from build123d import *

# Parameters (mm, degrees)
EXTRUDE_1_DEPTH          = 4
CUT_EXTRUDE_1_DEPTH      = 3
CUT_EXTRUDE_2_DEPTH      = 8.071067812
CUT_EXTRUDE_2_DEPTH_BACK = 3
SKETCH_4_R               = 1
CUT_EXTRUDE_3_DEPTH      = 3


with BuildPart() as part:
    # 草圖1 → 填料-伸長1 (new body)
    with BuildSketch(Plane(origin=(0, 0, 0), x_dir=(0, 0, -1), z_dir=(1, 0, 0))):
        with BuildLine():
            Line((0, 0), (-3, 0))
            Line((-3, 0), (-3, -4))
            ThreePointArc((-3, -4), (-2.707106781, -4.707106781), (-2, -5))
            Line((-2, -5), (2, -5))
            Line((2, -5), (2, -4))
            Line((2, -4), (-1, -4))
            ThreePointArc((-1, -4), (-1.707106781, -3.707106781), (-2, -3))
            Line((-2, -3), (-2, -1))
            Line((-2, -1), (0, -1))
            Line((0, -1), (0, 0))
        make_face()
    extrude(amount=EXTRUDE_1_DEPTH)

    # 草圖2 → 除料-伸長1 (cut)
    with BuildSketch(Plane(origin=(0, 0, 0), x_dir=(1, 0, 0), z_dir=(0, 1, 0))):
        with BuildLine():
            ThreePointArc((0, -1), (0.292893219, -0.292893219), (1, 0))
            Line((1, 0), (0, 0))
            Line((0, 0), (0, -1))
        make_face()
        with BuildLine():
            Line((4, 0), (3, 0))
            ThreePointArc((3, 0), (3.707106781, -0.292893219), (4, -1))
            Line((4, -1), (4, 0))
        make_face()
    extrude(amount=-CUT_EXTRUDE_1_DEPTH, mode=Mode.SUBTRACT)

    # 草圖3 → 除料-伸長2 (cut, two sides: drawn at the far end of the back side and taken through both)
    with BuildSketch(Plane.XZ.offset(5).offset(-CUT_EXTRUDE_2_DEPTH_BACK)):
        with BuildLine():
            Line((0, -0.361789115), (0, -2))
            Line((0, -2), (2, -2))
            ThreePointArc((2, -2), (0.585786438, -1.414213562), (0, 0))
            Line((0, 0), (0, -0.361789115))
        make_face()
        with BuildLine():
            ThreePointArc((4, 0), (3.414213562, -1.414213562), (2, -2))
            Line((2, -2), (4, -2))
            Line((4, -2), (4, -0.361789115))
            Line((4, -0.361789115), (4, 0))
        make_face()
    extrude(amount=CUT_EXTRUDE_2_DEPTH + CUT_EXTRUDE_2_DEPTH_BACK, mode=Mode.SUBTRACT)

    # 草圖4 → 除料-伸長3 (cut)
    with BuildSketch(Plane.XZ.offset(5)):
        with Locations(Location((2, 0, 0), (0, 0, 270))):
            Circle(SKETCH_4_R)
    extrude(amount=-CUT_EXTRUDE_3_DEPTH, mode=Mode.SUBTRACT)


solid = part.part
The model under review builds one solid part; all positions refer to its coordinate system, in mm. A direction names the side the tool comes from. Coordinates: 2 decimals unless noted, no trailing zeros. Write each loop counter-clockwise with the first axis right and the second up, starting at its lowest first coordinate (ties: lowest second). Pieces come first, ordered by that corner, then holes. Notation, with made-up numbers: (75, -30.5) -> (123, -30.5) arc R23 ccw to (123, 3.5) -> close; hole circle Ø9 at (70, 64). An arc over 180 degrees is marked (long way). Answer in a Markdown table with one row per item.
1. We need section A-A, the plane z = 1.55. State the section outline as (x, y) points, and give its area (3 significant figures).
Answers below:
| item | result |
|---|---|
| outline | (0, -5) -> (4, -5) -> (4, -3.84) -> (0, -3.84) -> close; (0, -1) -> (4, -1) -> (4, 0) -> (0, 0) -> close |
| area | 8.66 mm^2 |
2. For faces 5 (the cylindrical face through (3.699, -0.493, 0.285)), 6 (the flat face through (3, -5, 1)), 7 (the flat face through (2, -2, 2)), list the 3-axis set-ups (+Z, -Z, +X, -X, +Y, -Y) from which the entire face can be reached by the end or side of a thin tool; tool diameter is ignored.
Answers below:
| item | result |
|---|---|
| face 5 | -Z, +X, +Y |
| face 6 | +Z, -Z, +X, -X, -Y |
| face 7 | -Z, +X, -X |
3. Draft analysis for pull direction Z (two halves, no side actions). For faces 1 (the flat face through (2, -4, -1.2)), 2 (the cylindrical face through (1.024, -4.507, 0.217)), 3 (the flat face through (2, -2, 3)), 4 (the cylindrical face through (0.285, -0.493, 0.301)), state which applies: +Z half, -Z half, draft (parallel to the pull), parting line (faces both ways), or undercut.
Answers below:
| item | result |
|---|---|
| face 1 | draft |
| face 2 | undercut |
| face 3 | +Z half |
| face 4 | -Z half |
4. We need section C-C, the plane y = -0.8. State the section outline as (x, z) points.
Answers below:
| item | result |
|---|---|
| outline | (0, 1) arc R1 ccw to (1, 0) -> (3, 0) arc R1 ccw to (4, 1) -> (4, 3) -> (0, 3) -> close |
5. Wall thickness on probe 1 along X at (y, z) = (-4.75, 0); probe 2 along Z at (x, y) = (1.7, -2.2); probe 3 along Y at (x, z) = (1.4, -1.7): over which ranges is each line inside the solid? List them lowest first. Write a range as [from, to].
Answers below:
| item | result |
|---|---|
| probe 1 | x = [0, 1], [3, 4] |
| probe 2 | z = [2, 3] |
| probe 3 | y = [-5, -4] |
6. Clearance check with flat-ended pins moving along their axes: pin 1 Ø0.8 at (x, y) = (1.5, -0.5) entering from -Z; pin 2 Ø1.6 at (x, z) = (2, 0) entering from -Y. State where each tip first meets the part, or that it passes through.
Answers below:
| item | result |
|---|---|
| pin 1 | stops at z = 0 |
| pin 2 | stops at y = -1 |
7. We need section B-B, the plane x = 2.45. State the section outline as (y, z) points.
Answers below:
| item | result |
|---|---|
| outline | (-5, -1.95) -> (-4, -1.95) -> (-4, -0.89) -> (-5, -0.89) -> close; (-5, 0.89) -> (-4, 0.89) -> (-4, 1) arc R1 cw to (-3, 2) -> (-1, 2) -> (-1, 0) -> (0, 0) -> (0, 3) -> (-4, 3) arc R1 ccw to (-5, 2) -> close |
8. We need section D-D, the plane z = 0.8. State the section outline as (x, y) points, and give its area (3 significant figures).
Answers below:
| item | result |
|---|---|
| outline | (0, -5) -> (1.4, -5) -> (1.4, -4) -> (0, -4) -> close; (0.02, -1) -> (3.98, -1) -> (3.98, 0) -> (0.02, 0) -> close; (2.6, -5) -> (4, -5) -> (4, -4) -> (2.6, -4) -> close |
| area | 6.76 mm^2 |
